Here's how the part is built. I have some questions about the finished solid (model axes, mm). Round coordinates to 2 decimals unless told otherwise and drop trailing zeros. Loops run counter-clockwise (first coordinate to the right, second up) from the corner with the lowest first, then second, coordinate; pieces in that order, holes last. Notation, with made-up numbers: M -4.5,22.5 L 42.5,22.5 A25 cw 42.5,51.5 Z; hole C -1.5,79.5 d7. An arc over 180 degrees is marked long. Answer as a JSON object with one key per item and string values.
Autodesk Inventor part; units mm, degrees
ref_plane "YZ Plane" through (0, 0, 0) normal (1, 0, 0) x (0, 1, 0)
ref_plane "XZ Plane" through (0, 0, 0) normal (0, 1, 0) x (-1, 0, 0)
ref_plane "XY Plane" through (0, 0, 0) normal (0, 0, 1) x (1, 0, 0)
sketch "Sketch1" plane through (0, 0, 0) normal (1, 0, 0) x (0, 1, 0)
  line L0 (0, 0) -> (400, 0)
  line L1 (400, 0) -> (400, -400)
  line L2 (400, -400) -> (0, -400)
  line L3 (0, -400) -> (0, 0)
  line L4 (400, 0) -> (403, 0)
  line L5 (403, 0) -> (403, -80)
  line L6 (403, -80) -> (400, -80)
  line L7 (400, -400) -> (403, -400)
  line L8 (403, -400) -> (403, -320)
  line L9 (403, -320) -> (400, -320)
  line L10 (400, -160) -> (403, -160)
  line L11 (403, -160) -> (403, -240)
  line L12 (403, -240) -> (400, -240)
  line L13 (80, 0) -> (80, 3)
  line L14 (80, 3) -> (160, 3)
  line L15 (160, 3) -> (160, 0)
  line L16 (320, 0) -> (320, 3)
  line L17 (320, 3) -> (240, 3)
  line L18 (240, 3) -> (240, 0)
  line L19 (200, 0) -> (200, -400) construction
  line L20 (0, -200) -> (400, -200) construction
  line L21 (0, -400) -> (400, -400)
  line L22 (80, -400) -> (80, -403)
  line L23 (80, -403) -> (160, -403)
  line L24 (160, -403) -> (160, -400)
  line L25 (320, -400) -> (320, -403)
  line L26 (320, -403) -> (240, -403)
  line L27 (240, -403) -> (240, -400)
  line L28 (0, 0) -> (0, -400)
  line L29 (0, 0) -> (-3, 0)
  line L30 (-3, 0) -> (-3, -80)
  line L31 (-3, -80) -> (0, -80)
  line L32 (0, -400) -> (-3, -400)
  line L33 (-3, -400) -> (-3, -320)
  line L34 (-3, -320) -> (0, -320)
  line L35 (0, -160) -> (-3, -160)
  line L36 (-3, -160) -> (-3, -240)
  line L37 (-3, -240) -> (0, -240)
  line L38 (0, 0) -> (130, 0)
  line L39 (130, 0) -> (133, 0)
  line L40 (133, 0) -> (267, 0)
  line L41 (267, 0) -> (270, 0)
  line L42 (133, -80) -> (130, -80)
  line L43 (133, -80) -> (133, -160)
  line L44 (133, -160) -> (130, -160)
  line L45 (130, -320) -> (133, -320)
  line L46 (133, -320) -> (133, -240)
  line L47 (133, -240) -> (130, -240)
  line L48 (133, -80) -> (130, -80)
  line L49 (130, -80) -> (130, -160)
  line L50 (130, -320) -> (130, -240)
  line L51 (400, -200) -> (0, -200) construction
  line L52 (267, -80) -> (270, -80)
  line L53 (267, -80) -> (267, -160)
  line L54 (267, -160) -> (270, -160)
  line L55 (270, -320) -> (267, -320)
  line L56 (267, -320) -> (267, -240)
  line L57 (267, -240) -> (270, -240)
  line L58 (267, -80) -> (270, -80)
  line L59 (270, -80) -> (270, -160)
  line L60 (270, -320) -> (270, -240)
  dimension "d0" = 400
  dimension "d1" = 400
  dimension "d2" = 3
  dimension "d3" = 80
  dimension "d4" = 3
  dimension "d5" = 80
  dimension "d6" = 80
  dimension "d7" = 3
  dimension "d8" = 80
  dimension "d13" = 3
  dimension "d14" = 80
  dimension "d17" = 130
  dimension "d18" = 3
  dimension "d19" = 134
  dimension "d20" = 3
  dimension "d21" = 80
  dimension "d22" = 80
  dimension "d24" = 80
  dimension "d25" = 3
extrude "Extrusion1" add sketch "Sketch1" along normal blind 3
properties part number "Pared estanteria"
Item 1: I want a section at A-A on z = -290. List the corners of the cut face in (x, y) for me.
Solution:
{"outline": "M 0,0 L 3,0 L 3,130 L 0,130 Z; M 0,133 L 3,133 L 3,267 L 0,267 Z; M 0,270 L 3,270 L 3,400 L 0,400 Z"}
Item 2: If I drill on L1, parallel to Y at x = 2.1, z = -294; L2, parallel to Z at x = 1.8, y = 131.5; L3, parallel to Z at x = 1.4, y = 328, over which ranges is the centre line in solid material (lowest first)? Write a range as from..to.
Solution:
{"L1": "y = 0..130, 133..267, 270..400", "L2": "z = -403..-320, -240..-160, -80..3", "L3": "z = -400..0"}
Item 3: For P1, Ø1.5, axis at x = 1.5, y = 402, coming from the -Z side; P2, Ø1.5, axis at x = 2, z = -294.5, coming from the +Y side; P3, Ø0.9, axis at x = 1, y = 219.5, coming from the +Z side, each with a flat end and sliding along its axis, tell me the tip position at first contact or that it passes through.
Solution:
{"P1": "stops at z = -400", "P2": "stops at y = 400", "P3": "stops at z = 0"}
Item 4: I want a section at B-B on x = 0.5. Count the separate pieces of the cut face and the enclosed holes in it, plus the area to 3 significant figures.
Solution:
{"separate pieces": "1", "enclosed holes": "4", "area": "161,000 mm2"}
